Source: CAD feature listing. Evaluate the final solid. Frame: model axes, mm. A direction names the side the tool comes from. Give positions to 0.01 mm unless a question says otherwise; leave off trailing zeros. Order: outer loops, then holes, each group sorted by start corner. A loop starts at its lowest first (then second) coordinate and runs counter-clockwise, first axis right, second up. Notation, with made-up numbers: (89.5, -23) - (100.5, -23) arc R22 ccw to (100.5, -7) - close; hole circle Ø6 at (49, 82). An arc over 180 degrees is marked (long way). Use CSV: the item, a comma, the result in double quotes.
```python
from build123d import *

# Parameters (mm, degrees)
SKETCH1_W                  = 15.7
SKETCH1_H                  = 18
SKETCH1_W_2                = 12.7
SKETCH1_H_2                = 1.5
BOSS_EXTRUDE1_DEPTH        = 12
CUT_EXTRUDE1_START         = -10
CUT_EXTRUDE1_DEPTH         = 3.5
M4_CLEARANCE_HOLE2_D       = 4.8
M4_CLEARANCE_HOLE2_DEPTH   = 10
M4_CLEARANCE_HOLE2_TIP     = 1.442065486
M2_5_CLEARANCE_HOLE1_D     = 3.1
M2_5_CLEARANCE_HOLE1_DEPTH = 10
M2_5_CLEARANCE_HOLE1_TIP   = 0.931333959
CUT_EXTRUDE3_START         = -6
SKETCH9_R                  = 1.55
CUT_EXTRUDE3_DEPTH         = 1
SKETCH14_W                 = 15.7
SKETCH14_H                 = 2.5
CUT_EXTRUDE5_DEPTH         = 8
FILLET1_R                  = 1.25


with BuildPart() as part:
    # Sketch1 → Boss-Extrude1 (new body)
    with BuildSketch(Plane(origin=(0, 0, 0), x_dir=(1, 0, 0), z_dir=(0, 1, 0))):
        with Locations((0, -6.75)):
            Rectangle(SKETCH1_W, SKETCH1_H)
        Rectangle(SKETCH1_W_2, SKETCH1_H_2, mode=Mode.SUBTRACT)
    extrude(amount=BOSS_EXTRUDE1_DEPTH)

    # Sketch2 → Cut-Extrude1 (cut)
    with BuildSketch(Plane.XY.offset(15.75).offset(CUT_EXTRUDE1_START)):
        Polygon((3.6, 12), (-3.6, 12), (-3.6, 8.078460969), (0, 10.156921938), (3.6, 8.078460969), align=None)
        Polygon((-3.6, 3.921539031), (0, 1.843078062), (3.6, 3.921539031), (3.6, 8.078460969), (0, 10.156921938), (-3.6, 8.078460969), align=None)
    extrude(amount=-CUT_EXTRUDE1_DEPTH, mode=Mode.SUBTRACT)

    # M4 Clearance Hole2
    with Locations(Plane(origin=(0, 0, -2.25), x_dir=(-1, 0, 0), z_dir=(0, 0, -1))):
        with Locations((0, 6)):
            Hole(M4_CLEARANCE_HOLE2_D / 2, depth=M4_CLEARANCE_HOLE2_DEPTH)
            with Locations((0, 0, -(M4_CLEARANCE_HOLE2_DEPTH + M4_CLEARANCE_HOLE2_TIP / 2))):  # 118° drill point
                Cone(0, M4_CLEARANCE_HOLE2_D / 2, M4_CLEARANCE_HOLE2_TIP, mode=Mode.SUBTRACT)

    # M2.5 Clearance Hole1
    with Locations(Plane(origin=(0, 12, 0), x_dir=(1, 0, 0), z_dir=(0, 1, 0))):
        with Locations((3.75, -12), (-3.75, -12)):
            Hole(M2_5_CLEARANCE_HOLE1_D / 2, depth=M2_5_CLEARANCE_HOLE1_DEPTH)
            with Locations((0, 0, -(M2_5_CLEARANCE_HOLE1_DEPTH + M2_5_CLEARANCE_HOLE1_TIP / 2))):  # 118° drill point
                Cone(0, M2_5_CLEARANCE_HOLE1_D / 2, M2_5_CLEARANCE_HOLE1_TIP, mode=Mode.SUBTRACT)

    # Sketch9 → Cut-Extrude3 (cut, symmetric)
    # profile 1 of 4: a face of its own
    with BuildSketch(Plane(origin=(0, 12, 0), x_dir=(1, 0, 0), z_dir=(0, 1, 0)).offset(CUT_EXTRUDE3_START)):
        Polygon((-3.75, -15.0022214), (-6.35, -13.5011107), (-6.35, -15.75), (-1.15, -15.75), (-1.15, -13.5011107), align=None)
    # profile 2 of 4: a face of its own
    with BuildSketch(Plane(origin=(0, 12, 0), x_dir=(1, 0, 0), z_dir=(0, 1, 0)).offset(CUT_EXTRUDE3_START)):
        Polygon((-6.35, -13.5011107), (-3.75, -15.0022214), (-1.15, -13.5011107), (-1.15, -10.4988893), (-3.75, -8.9977786), (-6.35, -10.4988893), align=None)
        with Locations(Location((-3.75, -12, 0), (0, 0, 270))):
            Circle(SKETCH9_R, mode=Mode.SUBTRACT)
    # profile 3 of 4: a face of its own
    with BuildSketch(Plane(origin=(0, 12, 0), x_dir=(1, 0, 0), z_dir=(0, 1, 0)).offset(CUT_EXTRUDE3_START)):
        Polygon((1.15, -13.5011107), (1.15, -15.75), (6.35, -15.75), (6.35, -13.5011107), (3.75, -15.0022214), align=None)
    # profile 4 of 4: a face of its own
    with BuildSketch(Plane(origin=(0, 12, 0), x_dir=(1, 0, 0), z_dir=(0, 1, 0)).offset(CUT_EXTRUDE3_START)):
        Polygon((1.15, -13.5011107), (3.75, -15.0022214), (6.35, -13.5011107), (6.35, -10.4988893), (3.75, -8.9977786), (1.15, -10.4988893), align=None)
        with Locations(Location((3.75, -12, 0), (0, 0, 270))):
            Circle(SKETCH9_R, mode=Mode.SUBTRACT)
    extrude(amount=CUT_EXTRUDE3_DEPTH, both=True, mode=Mode.SUBTRACT)

    # Sketch14 → Cut-Extrude5 (cut)
    with BuildSketch(Plane.XY.offset(15.75)):
        with Locations((0, 1.25)):
            Rectangle(SKETCH14_W, SKETCH14_H)
        with Locations((0, 10.75)):
            Rectangle(SKETCH14_W, SKETCH14_H)
    extrude(amount=-CUT_EXTRUDE5_DEPTH, mode=Mode.SUBTRACT)

    # Fillet1
    fillet1_edges = [part.edges().sort_by_distance(p)[0] for p in [
        (7.85, 0, 2.75),
        (7.85, 12, 2.75),
        (-7.85, 12, 2.75),
        (-7.85, 0, 2.75),
    ]]
    fillet(fillet1_edges, radius=FILLET1_R)


solid = part.part
```
Item 1: Section A-A on z = 2. Return the cut outline in (x, y), then the cut area to 3 significant figures.
Filled in:
outline,"(-7.85, 1.25) arc R1.25 ccw to (-6.6, 0) - (6.6, 0) arc R1.25 ccw to (7.85, 1.25) - (7.85, 10.75) arc R1.25 ccw to (6.6, 12) - (-6.6, 12) arc R1.25 ccw to (-7.85, 10.75) - close; hole circle Ø4.8 at (0, 6)"
area,"169 mm2"
Item 2: Material intervals for line 1 (Z direction, x = 2, y = 4); line 2 (Z direction, x = 3.75, y = 7.6); line 3 (X direction, y = 3.95, z = 12), sorted ascending. Write a range as from..to.
Filled in:
line 1,"z = -2.25..-0.75, 0.75..2.25, 5.75..15.75"
line 2,"z = -2.25..-0.75, 0.75..10.45, 13.55..15.75"
line 3,"x = -7.85..-5.3, -2.2..2.2, 5.3..7.85"
Item 3: Mould query, pull axis X, two halves, no side actions, for faces 1 (the cylindrical face through (7.474, 11.644, 2.68)), 2 (the flat face through (0, 3, -2.25)), 3 (the conical face through (0.09, 5.59, 8.94)), 4 (the cylindrical face through (1.29, 8.024, -1.489)). Classes: released by +X, released by -X, zero draft, split by the parting line, or undercut.
Filled in:
face 1,"released by +X"
face 2,"zero draft"
face 3,"undercut"
face 4,"undercut"
Item 4: Section C-C on y = 1.5. Return the cut outline in (x, z), then the cut area to 3 significant figures.
Filled in:
outline,"(-7.85, -2.25) - (7.85, -2.25) - (7.85, 7.75) - (-7.85, 7.75) - close; hole (-6.35, -0.75) - (6.35, -0.75) - (6.35, 0.75) - (-6.35, 0.75) - close"
area,"138 mm2"
Item 5: Set-up query: faces 5 (the flat face through (0, 1, 7.75)), 6 (the cylindrical face through (1.29, 8.024, 6.764)), 7 (the flat face through (-5.032, 5.986, 9.738)). Return all of +Z, -Z, +X, -X, +Y, -Y with unobstructed straight access to the full face (end or side cutting, diameter ignored); none if empty.
Filled in:
face 5,"+Z, +X, -X, -Y"
face 6,"-Z"
face 7,"+Z"
Item 6: First-contact query: pin 1 (2.5 mm diameter, centred on x = -2.5, z = 14, fed in from +Y); pin 2 (3.5 mm diameter, centred on x = 0.5, y = 6, fed in from -Z); pin 3 (8 mm diameter, centred on x = 4.5, z = 12, fed in from -Y); pin 4 (3 mm diameter, centred on x = 3.75, z = 12, fed in from +Y). Flat tips, straight axial feed; report the tip coordinate or a pass-through.
Filled in:
pin 1,"stops at y = 9.5"
pin 2,"stops at z = 7.84"
pin 3,"stops at y = 2.5"
pin 4,"passes through"
Item 7: Section B-B on z = 12. Return the cut outline in (x, y).
Filled in:
outline,"(-7.85, 2.5) - (-5.3, 2.5) - (-5.3, 5) - (-6.35, 5) - (-6.35, 7) - (-5.3, 7) - (-5.3, 9.5) - (-7.85, 9.5) - close; (-2.2, 2.5) - (2.2, 2.5) - (2.2, 5) - (1.15, 5) - (1.15, 7) - (2.2, 7) - (2.2, 9.5) - (-2.2, 9.5) - (-2.2, 7) - (-1.15, 7) - (-1.15, 5) - (-2.2, 5) - close; (5.3, 2.5) - (7.85, 2.5) - (7.85, 9.5) - (5.3, 9.5) - (5.3, 7) - (6.35, 7) - (6.35, 5) - (5.3, 5) - close"
Item 8: Section D-D on z = 0. Return the cut outline in (x, y), then the cut area to 3 significant figures.
Filled in:
outline,"(-7.85, 1.25) arc R1.25 ccw to (-6.6, 0) - (-6.35, 0) - (-6.35, 12) - (-6.6, 12) arc R1.25 ccw to (-7.85, 10.75) - close; (6.35, 0) - (6.6, 0) arc R1.25 ccw to (7.85, 1.25) - (7.85, 10.75) arc R1.25 ccw to (6.6, 12) - (6.35, 12) - close"
area,"34.7 mm2"
